Geometry check sheet. Reference: drawing and pictorial views, mm from the part's lowest x, y, z. A direction names the side the tool comes from. Coordinates: 2 decimals unless noted, no trailing zeros. Loops run counter-clockwise (first coordinate to the right, second up) from the corner with the lowest first, then second, coordinate; pieces in that order, holes last. Notation, with made-up numbers: (57, 43.25) -> (70, 43.25) arc R12 cw to (70, 65.25) -> close; hole circle Ø4 at (18, 38.5). An arc over 180 degrees is marked (long way). Answer as a JSON object with one key per item and string values.
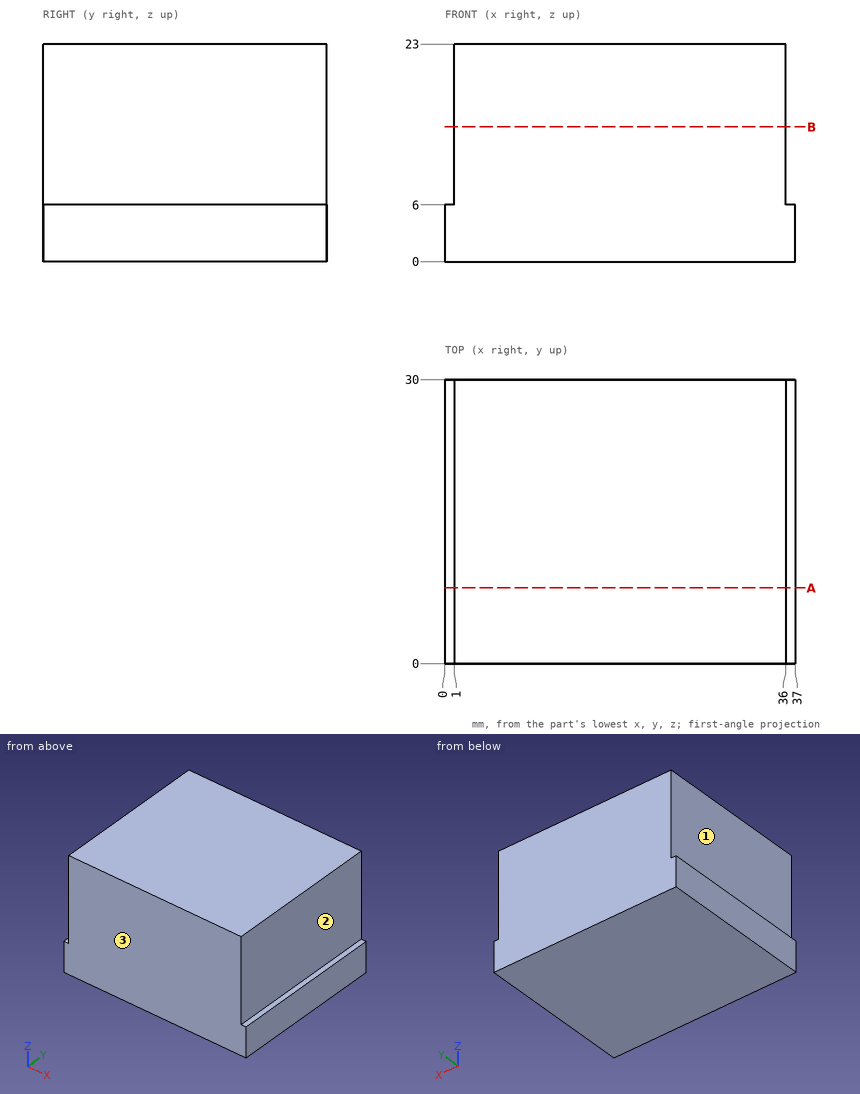
1. Depth check by flat-ended pin: P1, Ø6, axis at y = 24, z = 18, coming from the -X side; P2, Ø0.8, axis at x = 0.5, y = 17.5, coming from the +Z side; P3, Ø6, axis at y = 5, z = 19.5, coming from the +X side. Enter the tip coordinate at first touch or a pass-through.
Evaluation:
{"P1": "stops at x = 1", "P2": "stops at z = 6", "P3": "stops at x = 36"}
2. Tool access check on the marked faces 1, 2 and 3. Record the directions out of +Z, -Z, +X, -X, +Y, -Y that give a thin tool (end or side, any length) a straight path to the whole face; none if there is none.
Evaluation:
{"face 1": "+Z, -X, +Y, -Y", "face 2": "+Z, +X, +Y, -Y", "face 3": "+Z, -Z, +X, -X, -Y"}
3. Section check A-A, the plane y = 8. Record the boundary of the cut face in (x, z), then the cut area to 3 significant figures.
Evaluation:
{"outline": "(0, 0) -> (37, 0) -> (37, 6) -> (36, 6) -> (36, 23) -> (1, 23) -> (1, 6) -> (0, 6) -> close", "area": "817 mm^2"}
4. Section check B-B, the plane z = 14.25. Record the boundary of the cut face in (x, y).
Evaluation:
{"outline": "(1, 0) -> (36, 0) -> (36, 30) -> (1, 30) -> close"}
5. Thickness scan on probe 1 along X at (y, z) = (25.5, 16.75). Record the ranges inside material, lowest first. Write a range as from..to.
Evaluation:
{"probe 1": "x = 1..36"}
